Autodesk Inventor part; units mm, degrees
ref_plane "YZ Plane" through (0, 0, 0) normal (1, 0, 0) x (0, 1, 0)
ref_plane "XZ Plane" through (0, 0, 0) normal (0, 1, 0) x (-1, 0, 0)
ref_plane "XY Plane" through (0, 0, 0) normal (0, 0, 1) x (1, 0, 0)
sketch "Эскиз1" plane through (0, 0, 0) normal (0, 0, 1) x (1, 0, 0)
  circle A0 centre (0, 0) radius 12.5
  dimension "d0" = 25
extrude "Выдавливание1" add sketch "Эскиз1" along normal blind 3
sketch "Эскиз2" plane through (0, 0, 3) normal (0, 0, 1) x (1, 0, 0)
  circle A0 centre (0, 0) radius 7.5
  dimension "d3" = 15
extrude "Выдавливание2" add sketch "Эскиз2" along normal blind 5
sketch "Эскиз3" plane through (0, 0, 8) normal (0, 0, 1) x (1, 0, 0)
  circle A0 centre (0, 0) radius 18.85
  dimension "d6" = 37.7
extrude "Выдавливание3" add sketch "Эскиз3" along normal blind 21
sketch "Эскиз4" plane through (0, 0, 29) normal (0, 0, 1) x (1, 0, 0)
  circle A0 centre (0, 0) radius 5
  dimension "d9" = 10
extrude "Выдавливание4" add sketch "Эскиз4" along normal blind 6
chamfer "Фаска1" distance 6 angle 66 1 edges at (-5, 0, 29) measured on face at (4.9353, -0.8021, 33)
sketch "Эскиз5" plane through (0, 0, 35) normal (0, 0, 1) x (1, 0, 0)
  circle A0 centre (0, 0) radius 2.5
  dimension "d15" = 5
extrude "Выдавливание5" add sketch "Эскиз5" along normal blind 18
sketch "Эскиз6" plane through (0, 0, 0) normal (0, 0, -1) x (-1, 0, 0)
  circle A0 centre (0, 0) radius 9.5 construction
  circle A1 centre (0, 0) radius 12.5 construction
  line L0 (6.7175, -6.7175) -> (-6.7175, -6.7175) construction
  line L1 (-6.7175, -6.7175) -> (-6.7175, 6.7175) construction
  line L2 (-6.7175, 6.7175) -> (6.7175, 6.7175) construction
  line L3 (6.7175, 6.7175) -> (6.7175, -6.7175) construction
  line L4 (6.7175, -6.7175) -> (-6.7175, 6.7175) construction
  line L5 (-6.7175, -6.7175) -> (6.7175, 6.7175) construction
  circle A2 centre (6.7175, -6.7175) radius 1.5
  circle A3 centre (-6.7175, -6.7175) radius 1.5
  circle A4 centre (-6.7175, 6.7175) radius 1.5
  circle A5 centre (6.7175, 6.7175) radius 1.5
  dimension "d20" = 19
  dimension "d21" = 3
  dimension "d22" = 3
  dimension "d23" = 3
  dimension "d24" = 3
extrude "Выдавливание6" cut sketch "Эскиз6" against normal blind 5
properties part number "Двигатель 3115"
The model under review builds one solid part; all positions refer to its coordinate system, in mm. A direction names the side the tool comes from. Coordinates: 2 decimals unless noted, no trailing zeros. Write each loop counter-clockwise with the first axis right and the second up, starting at its lowest first coordinate (ties: lowest second). Pieces come first, ordered by that corner, then holes. Notation, with made-up numbers: (-8.5, 59.25) - (41.5, 59.25) arc R21 cw to (41.5, 73.25) - close; hole circle Ø3 at (83.25, -16.75). An arc over 180 degrees is marked (long way). Write item = value, one per line.
(1) Consider section D-D, the plane z = 38.5. Give the boundary of the cut face in (x, y), then the cut area to 3 significant figures.
Result sheet:
outline = circle Ø5 at (0, 0)
area = 19.6 mm^2
(2) Machinability: for faces 4 (the face through (-7.524, 7.982, 1.479)), 5 (the face through (8, 0, 8)), 6 (the face through (13.9, -12.5, 29)), which of the approach directions +Z, -Z, +X, -X, +Y, -Y give a long, thin tool a straight path to every point of the face, cutting with its end or side? Answer none if there is none.
Result sheet:
face_4 = -Z
face_5 = none
face_6 = +Z
(3) For line 1 (Z direction, x = 3, y = 2); line 2 (Z direction, x = -6.5, y = 6); line 3 (X direction, y = 13.5, z = 27.5), list the stretches that pass through material, from the lowest coordinate up. Write a range as [from, to].
Result sheet:
line_1 = [0, 35]
line_2 = [8, 33.29]
line_3 = [-13.16, 13.16]
(4) Consider section C-C, the plane z = 26. Give the boundary of the cut face in (x, y), then the cut area to 3 significant figures.
Result sheet:
outline = circle Ø37.7 at (0, 0)
area = 1,120 mm^2
(5) Mouldability with a two-part tool opening along Y and no side actions: class faces 1 (the face through (0, 0, 0)), 2 (the face through (-0.54, 2.44, 43.87)), 3 (the face through (5.287, -6.267, 1.479)) as pulls with the +Y half, pulls with the -Y half, needs draft (parallel to the pull), parting line crosses it, or undercut.
Result sheet:
face_1 = needs draft
face_2 = parting line crosses it
face_3 = undercut
(6) For P1, Ø2, axis at x = -14, z = 20, coming from the -Y side; P2, Ø2, axis at x = 0, z = 26, coming from the +Y side; P3, Ø12.5, axis at x = 1.5, y = -6, coming from the +Z side; P4, Ø10, axis at y = 8, z = 18.5, coming from the -X side, all flat-tipped, find the tip position at first contact; note any pin that passes through.
Result sheet:
P1 = -13.65
P2 = 18.85
P3 = 53
P4 = -18.61
